from build123d import *

# Parameters (mm, degrees)
SKETCH_1_R          = 1.6
SKETCH_1_R_2        = 6.075
EXTRUDE_1_DEPTH     = 4
CUT_EXTRUDE_1_REACH = 75.125
SKETCH_2_R          = 1.6
CUT_EXTRUDE_2_REACH = 75.125
SKETCH_3_R          = 1.6
CUT_EXTRUDE_3_REACH = 75.125
SKETCH_4_R          = 1.55
EXTRUDE_START       = -4
SKETCH_5_R          = 6.075
SKETCH_5_R_2        = 5.5
EXTRUDE_2_DEPTH     = 4
CHAMFER_1_SIZE      = 20
CUT_EXTRUDE_4_DEPTH = 10


with BuildPart() as part:
    # 草图1 → 凸台-拉伸1 (new body)
    with BuildSketch(Plane(origin=(0, 0, 0), x_dir=(-1, 0, 0), z_dir=(0, 0, -1))):
        with BuildLine():
            Line((12.5, 0), (12.5, 15))
            Line((12.5, 15), (12.5, 45))
            Line((12.5, 45), (-17.5, 45))
            Line((-17.5, 45), (-57.5, 45))
            Line((-57.5, 45), (-57.5, 13))
            Line((-57.5, 13), (-22.5, 13))
            ThreePointArc((-22.5, 13), (-15.428932188, 10.071067812), (-12.5, 3))
            Line((-12.5, 3), (-12.5, 0))
            ThreePointArc((-12.5, 0), (0, -12.5), (12.5, 0))
        make_face()
        with Locations(Location((-54.5, 19, 0), (0, 0, 180))):
            Circle(SKETCH_1_R, mode=Mode.SUBTRACT)
        with Locations(Location((-24.5, 19, 0), (0, 0, 180))):
            Circle(SKETCH_1_R, mode=Mode.SUBTRACT)
        with Locations(Location((-24.5, 39, 0), (0, 0, 180))):
            Circle(SKETCH_1_R, mode=Mode.SUBTRACT)
        with Locations(Location((-54.5, 39, 0), (0, 0, 180))):
            Circle(SKETCH_1_R, mode=Mode.SUBTRACT)
        with Locations(Location((0, 0, 0), (0, 0, 180))):
            Circle(SKETCH_1_R_2, mode=Mode.SUBTRACT)
    extrude(amount=-EXTRUDE_1_DEPTH)

    # 草图2 → 切除-拉伸1 (cut, up to next)
    with BuildSketch(Plane(origin=(0, 0, 0), x_dir=(-1, 0, 0), z_dir=(0, 0, -1)), mode=Mode.PRIVATE) as cut_extrude_1_sk1:
        with Locations((0, 10)):
            Circle(SKETCH_2_R)
    cut_extrude_1_tool1 = extrude(cut_extrude_1_sk1.sketch, amount=-CUT_EXTRUDE_1_REACH, mode=Mode.PRIVATE) & part.part
    add(cut_extrude_1_tool1.solids().sort_by_distance((0, 10, 0))[0], mode=Mode.SUBTRACT)

    # 草图3 → 切除-拉伸2 (cut, up to next)
    with BuildSketch(Plane.XY.offset(4), mode=Mode.PRIVATE) as cut_extrude_2_sk1:
        with Locations((10, 10)):
            Circle(SKETCH_3_R)
    cut_extrude_2_tool1 = extrude(cut_extrude_2_sk1.sketch, amount=-CUT_EXTRUDE_2_REACH, mode=Mode.PRIVATE) & part.part
    add(cut_extrude_2_tool1.solids().sort_by_distance((10, 10, 4))[0], mode=Mode.SUBTRACT)

    # 草图4 → 切除-拉伸3 (cut, up to next)
    with BuildSketch(Plane.XY.offset(4), mode=Mode.PRIVATE) as cut_extrude_3_sk1:
        with Locations((41.903612375, 19.168270074)):
            Circle(SKETCH_4_R)
    cut_extrude_3_tool1 = extrude(cut_extrude_3_sk1.sketch, amount=-CUT_EXTRUDE_3_REACH, mode=Mode.PRIVATE) & part.part
    add(cut_extrude_3_tool1.solids().sort_by_distance((41.903612, 19.16827, 4))[0], mode=Mode.SUBTRACT)

    # 草图5 → 凸台-拉伸2 (add)
    with BuildSketch(Plane.XY.offset(4).offset(EXTRUDE_START)):
        Circle(SKETCH_5_R)
        Circle(SKETCH_5_R_2, mode=Mode.SUBTRACT)
    extrude(amount=EXTRUDE_2_DEPTH)

    # 倒角1
    chamfer_1_edges = [part.edges().sort_by_distance(p)[0] for p in [
        (-12.5, 45, 2),
    ]]
    chamfer(chamfer_1_edges, length=CHAMFER_1_SIZE)

    # 草图6 → 切除-拉伸4 (cut)
    with BuildSketch(Plane.XY.offset(4)):
        with BuildLine():
            Line((9.634482471, 38.649201097), (2.113604897, 31.128323523))
            ThreePointArc((2.113604897, 31.128323523), (1.812829409, 28.685123781), (4.110129794, 27.800758579))
            Line((4.110129794, 27.800758579), (18.692042435, 32.238632926))
            ThreePointArc((18.692042435, 32.238632926), (20.106354196, 34.035811099), (18.910017796, 35.984889435))
            Line((18.910017796, 35.984889435), (11.848982729, 39.067892662))
            ThreePointArc((11.848982729, 39.067892662), (10.677142261, 39.200171443), (9.634482471, 38.649201097))
        make_face()
        with BuildLine():
            Line((32.71747005, 36.620860129), (42.227284145, 26.633201667))
            ThreePointArc((42.227284145, 26.633201667), (44.130956278, 26.064840044), (45.58542604, 27.418176749))
            Line((45.58542604, 27.418176749), (48.692879305, 37.405835211))
            ThreePointArc((48.692879305, 37.405835211), (48.393816721, 39.185679219), (46.783175609, 40))
            Line((46.783175609, 40), (34.165908249, 40))
            ThreePointArc((34.165908249, 40), (32.327664557, 38.787946781), (32.71747005, 36.620860129))
        make_face()
        with BuildLine():
            Line((-6.5, 18.908624945), (-6.5, 14.540152244))
            ThreePointArc((-6.5, 14.540152244), (-5.580990037, 12.857457816), (-3.668539461, 12.721176331))
            Line((-3.668539461, 12.721176331), (24.927936602, 25.79273008))
            ThreePointArc((24.927936602, 25.79273008), (25.966793038, 28.320165173), (23.514164728, 29.525057374))
            Line((23.514164728, 29.525057374), (-5.082311335, 20.821976327))
            ThreePointArc((-5.082311335, 20.821976327), (-6.106957166, 20.099292264), (-6.5, 18.908624945))
        make_face()
    extrude(amount=-CUT_EXTRUDE_4_DEPTH, mode=Mode.SUBTRACT)


solid = part.part
The model under review builds one solid part; all positions refer to its coordinate system, in mm. A direction names the side the tool comes from. Give positions to 0.01 mm unless a question says otherwise; leave off trailing zeros. Write each loop counter-clockwise with the first axis right and the second up, starting at its lowest first coordinate (ties: lowest second). Pieces come first, ordered by that corner, then holes. Notation, with made-up numbers: M -39.5,80.25 L 17.5,80.25 A26 cw 17.5,112.25 Z; hole C -16,88.5 d9. An arc over 180 degrees is marked long. One line per question, with ' | ' between items. Start each with the question number.
Item 1: We need section C-C on x = 0. Write out the cut boundary in (y, z), plus the area to 3 significant figures.
Item 2: We need section A-A on x = 54.5. Write out the cut boundary in (y, z), plus the area to 3 significant figures.
Item 3: We need section D-D on z = 0.95. Give the number of separate pieces and of enclosed holes in the cut face, plus the area to 3 significant figures.
Item 4: For faces 4 (the flat face through (12.5, 2, 2)), 5 (the flat face through (11.3, 29.99, 2.03)), 6 (the flat face through (-2.4, 35.1, 2)), list the 3-axis set-ups (+Z, -Z, +X, -X, +Y, -Y) from which the entire face can be reached by the end or side of a thin tool; tool diameter is ignored.
Item 5: For pin 1 (5 mm diameter, centred on x = 41.9, y = 19.17, fed in from -Z); pin 2 (2 mm diameter, centred on x = 39.5, z = 2.5, fed in from -Y), all flat-tipped, find the tip position at first contact; note any pin that passes through.
Item 6: We need section B-B on y = 16. Write out the cut boundary in (x, z).
Item 7: Wall thickness on line 1 (Y direction, x = 54.5, z = 0.9); line 2 (Y direction, x = 43.5, z = 3.35); line 3 (X direction, y = 39, z = 1): over which ranges is each line inside the solid? List them lowest first. Write a range as from..to.
Item 8: Draft analysis for pull direction Y (two halves, no side actions). For faces 1 (the cylindrical face through (15.51, 10.15, 1.97)), 2 (the cylindrical face through (55.36, 17.65, 1.97)), 3 (the flat face through (22, 23, 0)), state which applies: released by +Y, released by -Y, zero draft, split by the parting line, or undercut.
Results found:
1) outline: M -12.5,0 L -5.5,0 L -5.5,4 L -12.5,4 Z; M 5.5,0 L 8.4,0 L 8.4,4 L 5.5,4 Z; M 11.6,0 L 14.4,0 L 14.4,4 L 11.6,4 Z; M 22.37,0 L 37.5,0 L 37.5,4 L 22.37,4 Z | area: 111 mm2
2) outline: M 13,0 L 17.4,0 L 17.4,4 L 13,4 Z; M 20.6,0 L 37.4,0 L 37.4,4 L 20.6,4 Z; M 40.6,0 L 45,0 L 45,4 L 40.6,4 Z | area: 102 mm2
3) separate pieces: 1 | enclosed holes: 11 | area: 2,010 mm2
4) face 4: +Z, -Z, +X, -Y | face 5: +Z, -Z | face 6: +Z, -Z, -X, +Y
5) pin 1: stops at z = 0 | pin 2: stops at y = 13
6) outline: M -12.5,0 L -6.5,0 L -6.5,4 L -12.5,4 Z; M 3.5,0 L 57.5,0 L 57.5,4 L 3.5,4 Z
7) line 1: y = 13..17.4, 20.6..37.4, 40.6..45 | line 2: y = 13..26.02, 40..45 | line 3: x = 1.5..10.11, 12..22.9, 26.1..32.43, 48.52..52.9, 56.1..57.5
8) face 1: released by -Y | face 2: undercut | face 3: zero draft
